Build history of the part. All positions in model axes, mm. Face numbers are marked on the shaded views. Give positions to 0.01 mm unless a question says otherwise; leave off trailing zeros. Loops run counter-clockwise (first coordinate to the right, second up) from the corner with the lowest first, then second, coordinate; pieces in that order, holes last. Notation, with made-up numbers: M -39.75,43 L -3.75,43 A24 cw -3.75,80 Z; hole C 47,-31 d8. An arc over 180 degrees is marked long. Answer as a JSON object with one key per item and string values. Group by question number.
1. Drop flat-ended pins along their axis: pin 1 Ø1 at (x, y) = (8.5, 25.5) entering from -Z; pin 2 Ø10 at (x, z) = (11, -18) entering from +Y; pin 3 Ø4.5 at (x, z) = (10, -16.5) entering from +Y; pin 4 Ø10 at (x, z) = (14.5, -7) entering from +Y. Give the stop position or say it passes through.
2. Slice it at C-C (x = 10). List the corners of the cut face in (y, z).
3. Drill centre lines: line 1 along X through (y, z) = (-2.15, -16.5); line 2 along Y through (x, z) = (4.25, -5); line 3 along Z through (x, y) = (5, 12). Where is each one in solid material? Low to high. Write a range as [from, to].
4. Slice it at A-A (z = -16.5). List the corners of the cut face in (x, y).
5. Slice it at D-D (x = 2.5). List the corners of the cut face in (y, z).
6. Slice it at B-B (y = 16.5). List the corners of the cut face in (x, z).
7. Mould opens along Z. For the marked faces 1, 2 and 3 say: released by +Z, released by -Z, zero draft, split by the parting line, or undercut.
from build123d import *

# Parameters (mm, degrees)
BASE_FLANGE1_DEPTH = 20
CUT_EXTRUDE1_REACH = 50.877
SKETCH6_R          = 2.5
CUT_EXTRUDE2_REACH = 50.877
SKETCH7_R          = 2.5


# Sheet-metal steps are written as plain solids
with BuildPart() as part:
    # Sketch1 → Base-Flange1 (new body)
    with BuildSketch(Plane(origin=(0, 0, 0), x_dir=(0, 0, -1), z_dir=(1, 0, 0))):
        with BuildLine():
            Line((30, 0), (3, 0))
            ThreePointArc((3, 0), (0.878679656, 0.878679656), (0, 3))
            Line((0, 3), (0, 30))
            Line((0, 30), (-3, 30))
            Line((-3, 30), (-3, 3))
            ThreePointArc((-3, 3), (-1.242640687, -1.242640687), (3, -3))
            Line((3, -3), (30, -3))
            Line((30, -3), (30, 0))
        make_face()
    extrude(amount=BASE_FLANGE1_DEPTH)

    # Sketch6 → Cut-Extrude1 (cut, up to next)
    with BuildSketch(Plane.XZ.offset(3), mode=Mode.PRIVATE) as cut_extrude1_sk1:
        with Locations(Location((10, -16.5, 0), (0, 0, 270))):
            Circle(SKETCH6_R)
    cut_extrude1_tool1 = extrude(cut_extrude1_sk1.sketch, amount=-CUT_EXTRUDE1_REACH, mode=Mode.PRIVATE) & part.part
    add(cut_extrude1_tool1.solids().sort_by_distance((10, -3, -16.5))[0], mode=Mode.SUBTRACT)

    # Sketch7 → Cut-Extrude2 (cut, up to next)
    with BuildSketch(Plane.XY.offset(3), mode=Mode.PRIVATE) as cut_extrude2_sk1:
        with Locations((10, 16.5)):
            Circle(SKETCH7_R)
    cut_extrude2_tool1 = extrude(cut_extrude2_sk1.sketch, amount=-CUT_EXTRUDE2_REACH, mode=Mode.PRIVATE) & part.part
    add(cut_extrude2_tool1.solids().sort_by_distance((10, 16.5, 3))[0], mode=Mode.SUBTRACT)


solid = part.part
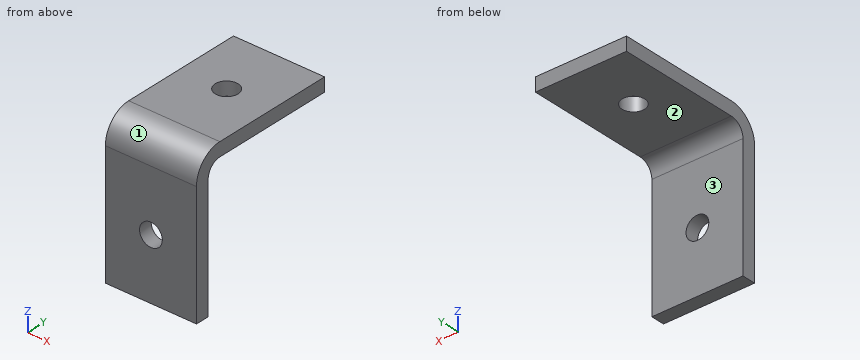
Established:
{
 "1": {"pin 1": "stops at z = 0", "pin 2": "stops at y = 0", "pin 3": "passes through", "pin 4": "stops at y = 0.17"},
 "2": {"outline": "M -3,-30 L 0,-30 L 0,-19 L -3,-19 Z; M -3,-14 L 0,-14 L 0,-3 A3 cw 3,0 L 14,0 L 14,3 L 3,3 A6 ccw -3,-3 Z; M 19,0 L 30,0 L 30,3 L 19,3 Z"},
 "3": {"line 1": "x = [0, 7.5], [12.5, 20]", "line 2": "y = [-3, 0]", "line 3": "z = [0, 3]"},
 "4": {"outline": "M 0,-3 L 7.5,-3 L 7.5,0 L 0,0 Z; M 12.5,-3 L 20,-3 L 20,0 L 12.5,0 Z"},
 "5": {"outline": "M -3,-30 L 0,-30 L 0,-3 A3 cw 3,0 L 30,0 L 30,3 L 3,3 A6 ccw -3,-3 Z"},
 "6": {"outline": "M 0,0 L 7.5,0 L 7.5,3 L 0,3 Z; M 12.5,0 L 20,0 L 20,3 L 12.5,3 Z"},
 "7": {"face 1": "released by +Z", "face 2": "released by -Z", "face 3": "zero draft"}
}
